from build123d import *

# Parameters (mm, degrees)
SKETCH1_W           = 21.5
SKETCH1_H           = 28.75
SKETCH1_W_2         = 13.5
SKETCH1_H_2         = 26.75
BOSS_EXTRUDE1_DEPTH = 1
SKETCH3_W           = 21.5
SKETCH3_H           = 12.5
BOSS_EXTRUDE2_DEPTH = 1
BOSS_EXTRUDE3_DEPTH = 2
BOSS_EXTRUDE4_START = -19.5
BOSS_EXTRUDE4_DEPTH = 2
BOSS_EXTRUDE5_REACH = 29.733
CUT_EXTRUDE1_DEPTH  = 23.460033949
SKETCH7_W           = 4
SKETCH7_H           = 28.75
BOSS_EXTRUDE8_DEPTH = 1
BOSS_EXTRUDE9_DEPTH = 0.5
FILLET2_R           = 74


with BuildPart() as part:
    # Sketch1 → Boss-Extrude1 (new body)
    with BuildSketch(Plane.XY):
        Rectangle(SKETCH1_W, SKETCH1_H)
        Rectangle(SKETCH1_W_2, SKETCH1_H_2, mode=Mode.SUBTRACT)
    extrude(amount=BOSS_EXTRUDE1_DEPTH)

    # Sketch3 → Boss-Extrude2 (add)
    with BuildSketch(Plane(origin=(0, 14.375, 0), x_dir=(1, 0, 0), z_dir=(0, 1, 0))):
        with Locations((0, -7.25)):
            Rectangle(SKETCH3_W, SKETCH3_H)
    extrude(amount=-BOSS_EXTRUDE2_DEPTH)

    # Sketch4 → Boss-Extrude3 (add)
    with BuildSketch(Plane(origin=(10.75, 0, 0), x_dir=(0, 0, -1), z_dir=(1, 0, 0))):
        with BuildLine():
            Line((-13.5, 13.375), (-13.5, 9.51786033))
            ThreePointArc((-13.5, 9.51786033), (-11.027421028, -3.345267641), (-3.962103479, -14.375))
            Line((-3.962103479, -14.375), (-1, -14.375))
            Line((-1, -14.375), (-1, 13.375))
            Line((-1, 13.375), (-13.5, 13.375))
        make_face()
    extrude(amount=-BOSS_EXTRUDE3_DEPTH)

    # Sketch4<2> → Boss-Extrude4 (add)
    with BuildSketch(Plane(origin=(10.75, 0, 0), x_dir=(0, 0, -1), z_dir=(1, 0, 0)).offset(BOSS_EXTRUDE4_START)):
        with BuildLine():
            Line((-13.5, 13.375), (-13.5, 9.51786033))
            ThreePointArc((-13.5, 9.51786033), (-11.027421028, -3.345267641), (-3.962103479, -14.375))
            Line((-3.962103479, -14.375), (-1, -14.375))
            Line((-1, -14.375), (-1, 13.375))
            Line((-1, 13.375), (-13.5, 13.375))
        make_face()
    extrude(amount=-BOSS_EXTRUDE4_DEPTH)

    # Sketch5 → Boss-Extrude5 (add, up to next)
    with BuildSketch(Plane.ZY.offset(-8.75), mode=Mode.PRIVATE) as boss_extrude5_sk1:
        with BuildLine():
            Line((12.5, 13.375), (13.5, 13.375))
            Line((13.5, 13.375), (13.5, 9.51786033))
            ThreePointArc((13.5, 9.51786033), (11.027421028, -3.345267641), (3.962103479, -14.375))
            Line((3.962103479, -14.375), (1, -14.375))
            Line((1, -14.375), (1, -13.104031722))
            ThreePointArc((1, -13.104031722), (9.459967949, -3.17071721), (12.5, 9.51786033))
            Line((12.5, 9.51786033), (12.5, 13.375))
        make_face()
    boss_extrude5_tool1 = extrude(boss_extrude5_sk1.sketch, amount=BOSS_EXTRUDE5_REACH, mode=Mode.PRIVATE) - part.part
    add(boss_extrude5_tool1.solids().sort_by_distance((8.75, -14.070646, 2.481052))[0])

    # Sketch6 → Cut-Extrude1 (cut, through all)
    with BuildSketch(Plane(origin=(0, 0, 0), x_dir=(-1, 0, 0), z_dir=(0, 0, -1))):
        Polygon((-6.75, 13.375), (6.75, 13.375), (6.75, 9.375), (-3.75, 9.375), (-3.75, 4.875), (-6.75, 4.875), align=None)
    extrude(amount=-CUT_EXTRUDE1_DEPTH, mode=Mode.SUBTRACT)

    # Sketch7 → Boss-Extrude8 (add)
    with BuildSketch(Plane(origin=(10.75, 0, 0), x_dir=(0, 0, -1), z_dir=(1, 0, 0))):
        with Locations((1, 0)):
            Rectangle(SKETCH7_W, SKETCH7_H)
    boss_extrude8 = extrude(amount=BOSS_EXTRUDE8_DEPTH)

    # Sketch7<5> → Boss-Extrude9 (add)
    with BuildSketch(Plane(origin=(10.75, 0, 0), x_dir=(0, 0, -1), z_dir=(1, 0, 0))):
        with BuildLine():
            Line((3, -10), (3, 10))
            ThreePointArc((3, 10), (2, 11), (1, 10))
            Line((1, 10), (1, -10))
            ThreePointArc((1, -10), (2, -11), (3, -10))
        make_face()
    boss_extrude9 = extrude(amount=-BOSS_EXTRUDE9_DEPTH)

    # Mirror3: Boss-Extrude8, Boss-Extrude9 across plane
    add(boss_extrude8.mirror(Plane(origin=(0, 0, 0), x_dir=(0, 0, 1), z_dir=(1, 0, 0))))
    add(boss_extrude9.mirror(Plane(origin=(0, 0, 0), x_dir=(0, 0, 1), z_dir=(1, 0, 0))))

    # Fillet2
    # the kernel refuses this fillet: 74 mm, written as the material it adds along each edge
    with BuildSketch(Plane(origin=(10.75, -14.375, 1), x_dir=(0, 0, 1), z_dir=(0, 1, 0))) as fillet2_piece_1_section:
        with BuildLine():
            CenterArc((12.124355653, 74), FILLET2_R, 260.569992092, 9.430007908)
            Line((0, 1), (0, 0))
            Line((0, 0), (12.124355653, 0))
        make_face()
    fillet2_piece_1 = extrude(amount=28.75, mode=Mode.PRIVATE)
    fillet2_piece_1 = fillet2_piece_1 & Plane(origin=(10.75, 9.51786033, -21.195293839), x_dir=(0, 0, 1), z_dir=(1, 0, 0)) * Cylinder(34.695293839, 106, mode=Mode.PRIVATE)
    add(fillet2_piece_1)
    with BuildSketch(Plane(origin=(-10.75, -14.375, 1), x_dir=(0, 0, 1), z_dir=(0, 1, 0))) as fillet2_piece_2_section:
        with BuildLine():
            CenterArc((12.124355653, -74), FILLET2_R, 90, 9.430007908)
            Line((0, -1), (0, 0))
            Line((0, 0), (12.124355653, 0))
        make_face()
    fillet2_piece_2 = extrude(amount=28.75, mode=Mode.PRIVATE)
    fillet2_piece_2 = fillet2_piece_2 & Plane(origin=(-10.75, 9.51786033, -21.195293839), x_dir=(0, 0, 1), z_dir=(1, 0, 0)) * Cylinder(34.695293839, 106, mode=Mode.PRIVATE)
    add(fillet2_piece_2)


solid = part.part
CAD build for the part. Positions are in the model's coordinates, mm. A direction names the side the tool comes from. Round coordinates to 2 decimals unless told otherwise and drop trailing zeros. Write each loop counter-clockwise with the first axis right and the second up, starting at its lowest first coordinate (ties: lowest second). Pieces come first, ordered by that corner, then holes.
(1) Mould opens along Z. For faces 1 (the face through (8, 11, 12.5)), 2 (the face through (-11.115, 2.993, 5.779)), 3 (the face through (-11, 0, -3)) say: pulls with the +Z half, pulls with the -Z half, needs draft (parallel to the pull), parting line crosses it, or undercut.
(2) Slice it at A-A, the plane z = -2. Write the cut outline in (x, y) (3 decimals), and give its area (3 significant figures).
(3) Drop flat-ended pins along their axis: P1, Ø1, axis at x = -6.5, y = -5.5, coming from the +Z side; P2, Ø8, axis at y = -4.5, z = 11, coming from the -X side; P3, Ø1.5, axis at x = 4, z = -1.5, coming from the +Y side; P4, Ø3, axis at y = 8.5, z = 11, coming from the +X side. Give the stop position or say it passes through.
(4) Slice it at C-C, the plane x = 7.5. Write the cut outline in (y, z) (3 decimals).
(5) Slice it at B-B, the plane x = -5. Write the cut outline in (y, z) (3 decimals), and give its area (3 significant figures).
(6) Slice it at D-D, the plane y = 6. Write the cut outline in (x, z).
(7) Probe line 1 along X through (y, z) = (-6, 0.25); line 2 along X through (y, z) = (8.25, 12.5); line 3 along Y through (x, z) = (-4.5, 10.25) (3 decimals). List the from-to ranges inside material, lowest first.
(8) 3-axis set-ups, long thin cutter, end or side, ignore diameter. For faces 4 (the face through (10.25, 0, -2)), 5 (the face through (-10.5, 11, -2)), 6 (the face through (10.5, -11, -2)), 7 (the face through (-6.75, 11, 13)), 8 (the face through (8, 0, 1)): which of +Z, -Z, +X, -X, +Y, -Y reach the whole face in a straight line?
From the geometry:
1. face 1: undercut
1. face 2: pulls with the +Z half
1. face 3: pulls with the -Z half
2. outline: (-11.75, -14.375) - (-10.75, -14.375) - (-10.75, -11) - (-10.25, -11) - (-10.25, 11) - (-10.75, 11) - (-10.75, 14.375) - (-11.75, 14.375) - close; (10.25, -11) - (10.75, -11) - (10.75, -14.375) - (11.75, -14.375) - (11.75, 14.375) - (10.75, 14.375) - (10.75, 11) - (10.25, 11) - close
2. area: 79.5 mm2
3. P1: stops at z = 10.32
3. P2: stops at x = -11
3. P3: passes through
3. P4: stops at x = 10.84
4. outline: (-14.375, 0) - (14.375, 0) - (14.375, 13.5) - (9.518, 13.5) arc R34.695 ccw to (-14.375, 3.962) - close; hole (-13.104, 1) - (13.375, 1) - (13.375, 12.5) - (9.518, 12.5) arc R28 ccw to start
5. outline: (-14.375, 0) - (-13.375, 0) - (-13.375, 1) - (-13.104, 1) arc R28 cw to (9.375, 12.5) - (9.375, 13.5) arc R34.695 ccw to (-14.375, 3.962) - close; (13.375, 0) - (14.375, 0) - (14.375, 13.5) - (13.375, 13.5) - close
5. area: 59.7 mm2
6. outline: (-11.75, -3) - (-10.25, -3) - (-10.25, -1) - (-10.75, -1) - (-10.75, 0) - (-6.75, 0) - (-6.75, 1) - (-8.75, 1) - (-8.75, 12.28) - (3.75, 12.28) - (3.75, 13.32) - (-10.75, 13.32) - (-10.75, 13.12) arc R74 cw to (-11.75, 1) - close; (6.75, 0) - (10.75, 0) - (10.75, -1) - (10.25, -1) - (10.25, -3) - (11.75, -3) - (11.75, 1) arc R74 cw to (10.75, 13.12) - (10.75, 13.32) - (6.75, 13.32) - (6.75, 12.28) - (8.75, 12.28) - (8.75, 1) - (6.75, 1) - close
7. line 1: x = -11.75 to -6.75, 6.75 to 11.75
7. line 2: x = -10.75 to 3.75, 6.75 to 10.75
7. line 3: y = -5.144 to -1.479, 13.375 to 14.375
8. face 4: -Z, +Y, -Y
8. face 5: +Y
8. face 6: -Y
8. face 7: +Z, -Z
8. face 8: none
